Autodesk Fusion 360 part; units mm, degrees
sketch "草图1" plane through (0, 0, 0) normal (0, 0, 1) x (1, 0, 0)
  line L0 (-125, 0) -> (125, 0) construction
  line L1 (0, -50) -> (0, 50) construction
  line L2 (-58, 0) -> (58, 0)
  line L3 (58, 30) -> (58, 0)
  line L4 (58, 30) -> (100, 30)
  line L5 (-58, 0) -> (-58, 30)
  line L6 (-58, 30) -> (-100, 30)
  circle A0 centre (-100, 72) radius 21
  circle A1 centre (100, 72) radius 21
  circle A2 centre (0, 42) radius 16
  line L7 (-100, 114) -> (-58, 114)
  line L8 (-58, 114) -> (-58, 144)
  line L9 (-58, 144) -> (58, 144)
  line L10 (58, 144) -> (58, 114)
  line L11 (58, 114) -> (100, 114)
  arc A3 (100, 30) -> (100, 114) centre (100, 72) ccw
  arc A4 (-100, 114) -> (-100, 30) centre (-100, 72) ccw
  line L12 (-58, 114) -> (-58, 30)
  line L13 (58, 114) -> (58, 30)
  dimension "d1" = 116
  dimension "d2" = 144
  dimension "d3" = 72
  dimension "d4" = 200
  dimension "d5" = 84
  dimension "d6" = 42
  dimension "d7" = 32
  dimension "d8" = 42
extrude "拉伸1" add sketch "草图1" along normal blind 32 contours L6 L7 A4 L12 | L4 L11 A3 L13 makes body 1 at (65, 72, 0) makes body 2 at (-65, 72, 0)
extrude "拉伸2" add sketch "草图1" along normal blind 48 contours L2 L3 L5 L8 L9 L10 L12 L13 bodies 1 2
sketch "草图2" plane through (-58, 0, 0) normal (-1, 0, 0) x (0, -1, 0)
  line L0 (-114, 0) -> (-114, 32)
  line L1 (-114, 32) -> (-30, 32)
  line L2 (-30, 32) -> (-30, 0)
  line L3 (-30, 0) -> (0, 0)
  line L4 (0, 0) -> (0, 48)
  line L5 (0, 48) -> (-144, 48)
  line L6 (-144, 48) -> (-144, 0)
  line L7 (-144, 0) -> (-114, 0)
  line L8 (-144, 48) -> (-144, 50)
  line L9 (-144, 50) -> (-144, 90)
  line L10 (-144, 90) -> (-124, 120)
  line L11 (-124, 120) -> (-96, 120)
  line L12 (-96, 120) -> (-96, 48)
  line L13 (-144, 48) -> (-96, 48)
  point P0 (-144, 0)
  dimension "d13" = 20
  dimension "d14" = 30
  dimension "d15" = 96
  dimension "d16" = 120
extrude "拉伸3" add sketch "草图2" against normal blind 116 contours L5 L8 L9 L10 L11 L12 L13 bodies 1
sketch "草图3" plane through (0, 0, 120) normal (0, 0, 1) x (-1, 0, 0)
  line L0 (58, -124) -> (58, -96)
  line L1 (58, -96) -> (-58, -96)
  line L2 (-58, -96) -> (-58, -124)
  line L3 (-58, -124) -> (58, -124)
  line L4 (0, -180) -> (0, 50) construction
  line L5 (58, -96) -> (58, -35)
  line L6 (58, -35) -> (33, 0)
  line L7 (33, 0) -> (-33, 0)
  line L8 (-33, 0) -> (-58, -35)
  line L9 (-58, -35) -> (-58, -96)
  line L10 (58, -96) -> (-58, -96)
  circle A0 centre (0, -42) radius 27
  circle A1 centre (0, -42) radius 16
  line L11 (100, 0) -> (-125.4385, 0) construction
  dimension "d19" = 116
  dimension "d20" = 66
  dimension "d21" = 35
  dimension "d22" = 54
  dimension "d23" = 32
  dimension "d25" = 42
extrude "拉伸4" add sketch "草图3" against normal blind 32 contours L1 L5 L6 L7 L8 L9 L10 | A0 bodies 1
extrude "拉伸5" cut sketch "草图3" against normal blind 22 contours A0 bodies 1
equation "d5 = ( 42 * 2 ) * 1 mm"
Work out the finished part from the listing and answer in its coordinate system (mm). A direction names the side the tool comes from. Round coordinates to 2 decimals unless told otherwise and drop trailing zeros. Loops run counter-clockwise (first coordinate to the right, second up) from the corner with the lowest first, then second, coordinate; pieces in that order, holes last. Notation, with made-up numbers: M 41.25,54.25 L 72.25,54.25 A17 ccw 72.25,66.25 Z; hole C -27.5,21.5 d6. An arc over 180 degrees is marked long. Use CSV: the item, a comma, the result in double quotes.
Q1. Section B-B, the plane z = 15 is taken. Determine the outline of the cut face in (x, y), then the cut area to 3 significant figures.
Determined:
outline,"M -100,30 L -58,30 L -58,0 L 58,0 L 58,30 L 100,30 A42 ccw 100,114 L 58,114 L 58,144 L -58,144 L -58,114 L -100,114 A42 ccw Z; hole C -100,72 d42; hole C 0,42 d32; hole C 100,72 d42"
area,"25,700 mm2"
Q2. Section D-D, the plane x = 107.5 is taken. Determine the outline of the cut face in (y, z).
Determined:
outline,"M 30.68,0 L 52.38,0 L 52.38,32 L 30.68,32 Z; M 91.62,0 L 113.32,0 L 113.32,32 L 91.62,32 Z"
Q3. The mould has two halves that part along Z. Classify faces 1 (the flat face through (-12, 58, 88)), 2 (the flat face through (-2, 73, 0)), 3 (the cylindrical face through (-12.459, 65.954, 109.154)), 4 (the flat face through (-1, 59, 48)): pulls with the +Z half, pulls with the -Z half, needs draft (parallel to the pull), parting line crosses it, or undercut.
Determined:
face 1,"undercut"
face 2,"pulls with the -Z half"
face 3,"needs draft"
face 4,"undercut"
Q4. Section C-C, the plane y = 42 is taken. Determine the outline of the cut face in (x, z), then the cut area to 3 significant figures.
Determined:
outline,"M -129.39,0 L -16,0 L -16,48 L -58,48 L -58,32 L -129.39,32 Z; M -58,88 L -16,88 L -16,98 L -27,98 L -27,120 L -58,120 Z; M 16,0 L 129.39,0 L 129.39,32 L 58,32 L 58,48 L 16,48 Z; M 16,88 L 58,88 L 58,120 L 27,120 L 27,98 L 16,98 Z"
area,"10,800 mm2"
Q5. Consider L1, parallel to Z at x = 27.5, y = 74; L2, parallel to Y at x = 100, z = 19; L3, parallel to Y at x = 0, z = 20.5. Determine where each line is inside the solid, lowest interval first.
Determined:
L1,"0 to 48, 88 to 120"
L2,"30 to 51, 93 to 114"
L3,"0 to 26, 58 to 144"
Q6. A tool of negligible diameter and unlimited length cuts with its end or side. For faces 5 (the flat face through (45.325, 17.255, 104.224)), 6 (the flat face through (-12, 54, 98)), 7 (the flat face through (-45.675, 17.745, 104.224)), from which of +Z, -Z, +X, -X, +Y, -Y can it reach the whole face along a straight path? Write none if from no direction.
Determined:
face 5,"+Z, +X, -Y"
face 6,"+Z"
face 7,"+Z, -X, -Y"
Q7. Each of these flat-tipped pins is pushed along its axis until it touches: pin 1 (6 mm diameter, centred on y = 119, z = 93.5, fed in from +X); pin 2 (9.5 mm diameter, centred on x = 84.5, z = 14, fed in from -Y); pin 3 (25 mm diameter, centred on x = -104, y = 53.5, fed in from +Z). Where does it stop, or does it pass through?
Determined:
pin 1,"x = 58"
pin 2,"y = 30"
pin 3,"z = 32"
Q8. Section A-A, the plane x = 0 is taken. Determine the outline of the cut face in (y, z).
Determined:
outline,"M 0,0 L 26,0 L 26,48 L 0,48 Z; M 0,88 L 26,88 L 26,98 L 15,98 L 15,120 L 0,120 Z; M 58,0 L 144,0 L 144,90 L 124,120 L 69,120 L 69,98 L 58,98 L 58,88 L 96,88 L 96,48 L 58,48 Z"
